```python
from build123d import *

# Parameters (mm, degrees)
SKETCH_1_W                  = 18
SKETCH_1_H                  = 18.5
EXTRUDE_1_DEPTH             = 1.5
SKETCH_2_W                  = 2
SKETCH_2_H                  = 18.5
EXTRUDE_2_DEPTH             = 18
SKETCH_5_W                  = 18
SKETCH_5_H                  = 1.5
EXTRUDE_5_DEPTH             = 15
SKETCH_6_R                  = 1
CUT_EXTRUDE_1_DEPTH         = 21.169593452
SKETCH_7_W                  = 14
SKETCH_7_H                  = 1.5
CUT_EXTRUDE_2_DEPTH         = 1
SKETCH_8_W                  = 27.6
SKETCH_8_H                  = 28.1
SKETCH_8_W_2                = 17.6
SKETCH_8_H_2                = 18.1
CUT_EXTRUDE_3_DEPTH         = 23.148645557
SKETCH_4_W                  = 5
SKETCH_4_H                  = 3
EXTRUDE_4_DEPTH             = 1.5
EXTRUDE_4_DIRECTION_2_REACH = 28.884
FILLET_1_R                  = 0.4


with BuildPart() as part:
    # Эскиз1 → Бобышка-Вытянуть1 (new body)
    with BuildSketch(Plane.XY):
        Rectangle(SKETCH_1_W, SKETCH_1_H)
        with BuildLine():
            Line((3.1, -2.197726098), (3.1, 2.197726098))
            ThreePointArc((3.1, 2.197726098), (0, 3.8), (-3.1, 2.197726098))
            Line((-3.1, 2.197726098), (-3.1, -2.197726098))
            ThreePointArc((-3.1, -2.197726098), (0, -3.8), (3.1, -2.197726098))
        make_face(mode=Mode.SUBTRACT)
    extrude(amount=-EXTRUDE_1_DEPTH)

    # Эскиз2 → Бобышка-Вытянуть2 (add)
    with BuildSketch(Plane.XY):
        with Locations((-8, 0)):
            Rectangle(SKETCH_2_W, SKETCH_2_H)
        with Locations((8, 0)):
            Rectangle(SKETCH_2_W, SKETCH_2_H)
    extrude(amount=-EXTRUDE_2_DEPTH)

    # Эскиз5 → Бобышка-Вытянуть5 (add)
    with BuildSketch(Plane(origin=(0, 9.25, 0), x_dir=(1, 0, 0), z_dir=(0, 1, 0))):
        with Locations((0, 16.25)):
            Rectangle(SKETCH_5_W, SKETCH_5_H)
    extrude(amount=-EXTRUDE_5_DEPTH)

    # Эскиз6 → Вырез-Вытянуть1 (cut, through all)
    with BuildSketch(Plane(origin=(0, 0, -15.5), x_dir=(-1, 0, 0), z_dir=(0, 0, -1))):
        with Locations((0, 2.5)):
            Circle(SKETCH_6_R)
        with Locations((0, -2.5)):
            Circle(SKETCH_6_R)
    extrude(amount=CUT_EXTRUDE_1_DEPTH, mode=Mode.SUBTRACT)

    # Эскиз7 → Вырез-Вытянуть2 (cut)
    with BuildSketch(Plane.XZ.offset(9.25)):
        with Locations((0, -0.75)):
            Rectangle(SKETCH_7_W, SKETCH_7_H)
    extrude(amount=-CUT_EXTRUDE_2_DEPTH, mode=Mode.SUBTRACT)

    # Эскиз8 → Вырез-Вытянуть3 (cut, through all)
    with BuildSketch(Plane.XY):
        Rectangle(SKETCH_8_W, SKETCH_8_H)
        Rectangle(SKETCH_8_W_2, SKETCH_8_H_2, mode=Mode.SUBTRACT)
    extrude(amount=-CUT_EXTRUDE_3_DEPTH, mode=Mode.SUBTRACT)

    # Эскиз4 → Бобышка-Вытянуть4 (add)
    with BuildSketch(Plane.ZY.offset(9)):
        with Locations((-9, 0)):
            Rectangle(SKETCH_4_W, SKETCH_4_H)
    extrude(amount=EXTRUDE_4_DEPTH)

    # Эскиз4 → Бобышка-Вытянуть4 direction 2 (add, up to next)
    with BuildSketch(Plane.ZY.offset(9), mode=Mode.PRIVATE) as extrude_4_direction_2_sk1:
        with Locations((-9, 0)):
            Rectangle(SKETCH_4_W, SKETCH_4_H)
    extrude_4_direction_2_tool1 = extrude(extrude_4_direction_2_sk1.sketch, amount=-EXTRUDE_4_DIRECTION_2_REACH, mode=Mode.PRIVATE) - part.part
    add(extrude_4_direction_2_tool1.solids().sort_by_distance((-9, 0, -9))[0])

    # Скругление1
    fillet_1_edges = [part.edges().sort_by_distance(p)[0] for p in [
        (-10.5, 0, -11.5),
        (-10.5, 0, -6.5),
    ]]
    fillet(fillet_1_edges, radius=FILLET_1_R)


solid = part.part
```
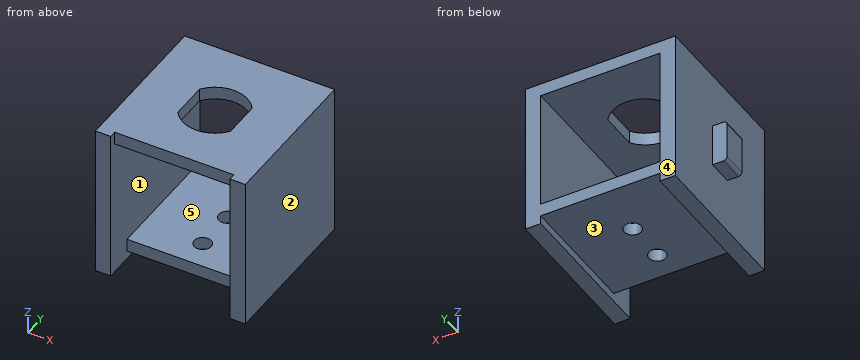
Input: part model. Units: mm. Frame: model coordinates. Face numbers are marked on the shaded views. A direction names the side the tool comes from. Coordinates: 2 decimals unless noted, no trailing zeros. Write each loop counter-clockwise with the first axis right and the second up, starting at its lowest first coordinate (ties: lowest second). Pieces come first, ordered by that corner, then holes. Notation, with made-up numbers: M -16.75,3 L 17.25,3 A30 ccw 17.25,37 Z; hole C 75,65 d8. An arc over 180 degrees is marked long. Use one line per item in the form item = value.
Q1. Section C-C (y = 4.5). Return loops of the section in (x, z), plus the area to 3 significant figures.
Answer below:
outline = M -8.8,-18 L -7,-18 L -7,-17 L 7,-17 L 7,-18 L 8.8,-18 L 8.8,0 L -8.8,0 Z; hole M -7,-15.5 L 7,-15.5 L 7,-1.5 L -7,-1.5 Z
area = 107 mm²
Q2. Section B-B (x = 0). Return loops of the section in (y, z), plus the area to 4 significant figures.
Answer below:
outline = M -8.25,-1.5 L -3.8,-1.5 L -3.8,0 L -8.25,0 Z; M -5.75,-17 L -3.5,-17 L -3.5,-15.5 L -5.75,-15.5 Z; M -1.5,-17 L 1.5,-17 L 1.5,-15.5 L -1.5,-15.5 Z; M 3.5,-17 L 9.05,-17 L 9.05,-15.5 L 3.5,-15.5 Z; M 3.8,-1.5 L 9.05,-1.5 L 9.05,0 L 3.8,0 Z
area = 30.75 mm²
Q3. Material intervals for probe 1 along Y at (x, z) = (0, -16.6); probe 2 along X at (y, z) = (-4.75, -2.5); probe 3 along Z at (x, y) = (-5, -1.5), sorted ascending. Write a range as from..to.
Answer below:
probe_1 = -5.75..-3.5, -1.5..1.5, 3.5..9.05
probe_2 = -8.8..-7, 7..8.8
probe_3 = -17..-15.5, -1.5..0
Q4. Section A-A (z = -2.5). Return loops of the section in (x, y), plus the area to 3 significant figures.
Answer below:
outline = M -8.8,-9.05 L -7,-9.05 L -7,9.05 L -8.8,9.05 Z; M 7,-9.05 L 8.8,-9.05 L 8.8,9.05 L 7,9.05 Z
area = 65.2 mm²
Q5. Draft query along Z for the marked faces 1, 2 and 3. Return one class per face: released by +Z, released by -Z, zero draft, split by the parting line, or undercut.
Answer below:
face_1 = undercut
face_2 = zero draft
face_3 = released by -Z
Q6. Section D-D (x = -4). Return loops of the section in (y, z), plus the area to 4 significant figures.
Answer below:
outline = M -8.25,-1.5 L 9.05,-1.5 L 9.05,0 L -8.25,0 Z; M -5.75,-17 L 9.05,-17 L 9.05,-15.5 L -5.75,-15.5 Z
area = 48.15 mm²
Q7. First-contact query: pin 1 (6 mm diameter, centred on x = -0.5, y = -7, fed in from -Z); pin 2 (5.5 mm diameter, centred on y = -4, z = -7.5, fed in from -X); pin 3 (0.8 mm diameter, centred on x = -0.5, z = -16.5, fed in from -Y); pin 4 (0.8 mm diameter, centred on x = -10, z = -8, fed in from +Y). Flat tips, straight axial feed; report the tip coordinate or a pass-through.
Answer below:
pin_1 = -17
pin_2 = -10.5
pin_3 = -5.75
pin_4 = 1.5
Q8. Set-up query: the marked faces 4 and 5. Return all of +Z, -Z, +X, -X, +Y, -Y with unobstructed straight access to the full face (end or side cutting, diameter ignored); none if empty.
Answer below:
face_4 = +Z, -Z, +X, -X, +Y
face_5 = +Y, -Y
